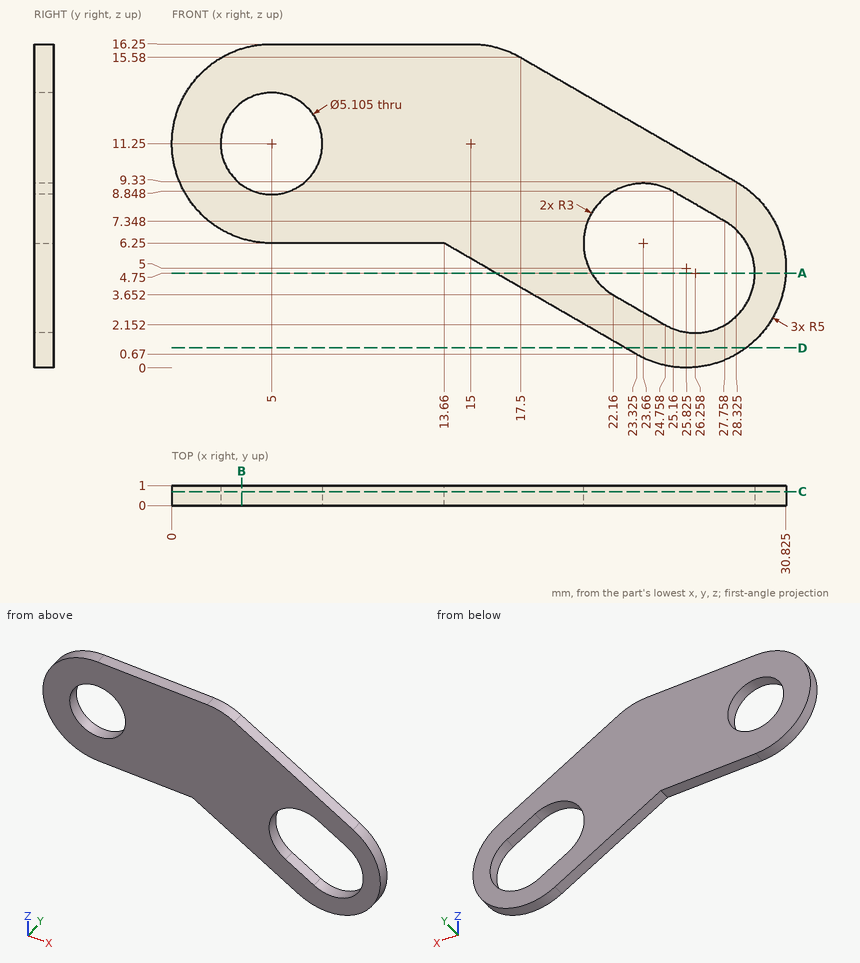
Here's the drawing with two shaded views (mm, measured from the low corner). I have some questions. Coordinates: 2 decimals unless noted, no trailing zeros. Write each loop counter-clockwise with the first axis right and the second up, starting at its lowest first coordinate (ties: lowest second). Pieces come first, ordered by that corner, then holes.
Item 1: I want a section at C-C on y = 0.7. Count the separate pieces of the cut face and the enclosed holes in it, and give its area (3 significant figures).
Item 2: Will these pins go through, and if not, where does the flat tip stop? pin 1 (1.5 mm diameter, centred on x = 13, z = 4.5, fed in from +Y); pin 2 (8 mm diameter, centred on x = 6, z = 3, fed in from +Y).
Item 3: I want a section at D-D on z = 1. Write out the boundary of the cut face in (x, y) (1 decimal).
Item 4: I want a section at A-A on z = 4.75. Write out the boundary of the cut face in (x, y).
Item 5: If I drill on line 1 (Z direction, x = 5, y = 0.2); line 2 (Z direction, x = 9, y = 0.25); line 3 (Z direction, x = 27, y = 0.55) (1 decimal), over which ranges is the centre line in solid material (lowest first)?
Item 6: I want a section at B-B on x = 3.5. Write out the boundary of the cut face in (y, z) (1 decimal).
Findings below:
1. separate pieces: 1
1. enclosed holes: 2
1. area: 237 mm2
2. pin 1: passes through
2. pin 2: stops at y = 1
3. outline: (22.8, 0) - (28.8, 0) - (28.8, 1) - (22.8, 1) - close
4. outline: (16.26, 0) - (21.06, 0) - (21.06, 1) - (16.26, 1) - close; (29.26, 0) - (30.82, 0) - (30.82, 1) - (29.26, 1) - close
5. line 1: z = 6.25 to 8.7, 13.8 to 16.25
5. line 2: z = 6.25 to 16.25
5. line 3: z = 0.1 to 1.8, 7.8 to 10.1
6. outline: (0, 6.5) - (1, 6.5) - (1, 9.2) - (0, 9.2) - close; (0, 13.3) - (1, 13.3) - (1, 16) - (0, 16) - close
